Read the model definition and answer for the solid it produces. Units are mm, in the model's axes. Face numbers are marked on the shaded views. A direction names the side the tool comes from. Round coordinates to 2 decimals unless told otherwise and drop trailing zeros. Order: outer loops, then holes, each group sorted by start corner. A loop starts at its lowest first (then second) coordinate and runs counter-clockwise, first axis right, second up. Notation, with made-up numbers: (-5, 74) - (29, 74) arc R22 ccw to (29, 88) - close; hole circle Ø11 at (-8, 29.5). An arc over 180 degrees is marked (long way). One line per question, with ' | ' between items. Start each with the question number.
1) The part is cut by section A-A, the plane y = 0. Give the vertices of the cut face in (x, z), plus the area to 3 significant figures.
2) The mould has two halves that part along Y. Classify the marked faces 3, 4 and 5: pulls with the +Y half, pulls with the -Y half, needs draft (parallel to the pull), parting line crosses it, or undercut.
3) For the marked faces 1 and 2, determine the directions among +Z, -Z, +X, -X, +Y, -Y from which every point of the face is accessible in a straight line to the end or side of a thin tool.
4) The part is cut by section C-C, the plane y = -25. Give the vertices of the cut face in (x, z).
5) Straight lines are drawn through the part: line 1 (Y direction, x = 0, z = -10.75); line 2 (Y direction, x = -26.5, z = -16.5). For each, find the intervals that lie inside material, in ascending order. Write a range as from..to.
6) The part is cut by section B-B, the plane z = -14. Give the vertices of the cut face in (x, y), plus the area to 3 significant figures.
from build123d import *

# Parameters (mm, degrees)
ESQUISSE1_W                  = 70
ESQUISSE1_H                  = 70
BOSS_EXTRU_1_DEPTH           = 20
ENL_V_MAT_EXTRU_1_DEPTH      = 54.38539126
ENL_V_MAT_EXTRU_1_DEPTH_BACK = 15
ESQUISSE2_R                  = 26
ESQUISSE3_R                  = 3
ENL_V_MAT_EXTRU_2_DEPTH      = 54.38539126


with BuildPart() as part:
    # Esquisse1 → Boss.-Extru.1 (new body)
    with BuildSketch(Plane.XY):
        Rectangle(ESQUISSE1_W, ESQUISSE1_H)
    extrude(amount=-BOSS_EXTRU_1_DEPTH)

    # Esquisse2 → Enlèv. mat.-Extru.1 (cut, two sides: drawn at the far end of the back side and taken through both)
    with BuildSketch(Plane.XY.offset(-ENL_V_MAT_EXTRU_1_DEPTH_BACK)):
        Circle(ESQUISSE2_R)
    extrude(amount=ENL_V_MAT_EXTRU_1_DEPTH + ENL_V_MAT_EXTRU_1_DEPTH_BACK, mode=Mode.SUBTRACT)

    # Esquisse3 → Enlèv. mat.-Extru.2 (cut, through all)
    with BuildSketch(Plane(origin=(0, 0, -20), x_dir=(-1, 0, 0), z_dir=(0, 0, -1))):
        with Locations((-25, 25)):
            Circle(ESQUISSE3_R)
        with Locations((25, 25)):
            Circle(ESQUISSE3_R)
        with Locations((25, -25)):
            Circle(ESQUISSE3_R)
        with Locations((-25, -25)):
            Circle(ESQUISSE3_R)
    extrude(amount=-ENL_V_MAT_EXTRU_2_DEPTH, mode=Mode.SUBTRACT)


solid = part.part
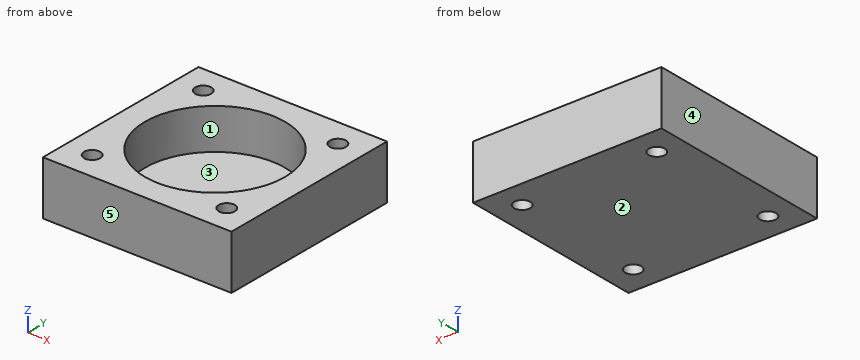
Values:
1) outline: (-35, -20) - (35, -20) - (35, 0) - (26, 0) - (26, -15) - (-26, -15) - (-26, 0) - (-35, 0) - close | area: 620 mm^2
2) face 3: undercut | face 4: needs draft | face 5: pulls with the -Y half
3) face 1: +Z | face 2: -Z, +X, -X, +Y, -Y
4) outline: (-35, -20) - (-28, -20) - (-28, 0) - (-35, 0) - close; (-22, -20) - (22, -20) - (22, 0) - (7.14, 0) - (7.14, -15) - (-7.14, -15) - (-7.14, 0) - (-22, 0) - close; (28, -20) - (35, -20) - (35, 0) - (28, 0) - close
5) line 1: y = -35..-26, 26..35 | line 2: y = -35..-27.6, -22.4..22.4, 27.6..35
6) outline: (-35, -35) - (35, -35) - (35, 35) - (-35, 35) - close; hole circle Ø6 at (-25, -25); hole circle Ø6 at (-25, 25); hole circle Ø52 at (0, 0); hole circle Ø6 at (25, -25); hole circle Ø6 at (25, 25) | area: 2,660 mm^2
